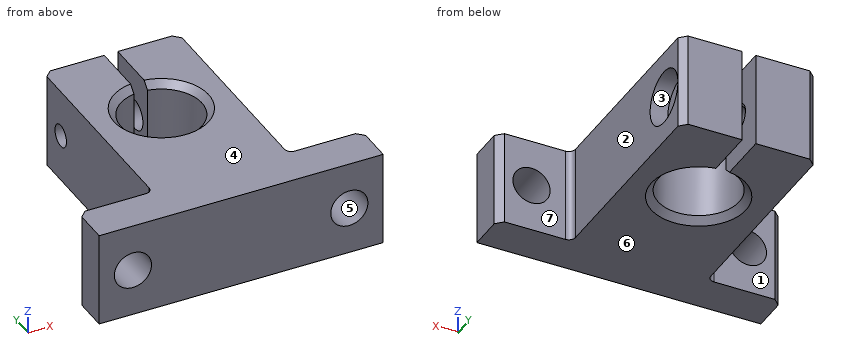
```python
from build123d import *

# Parameters (mm, degrees)
ESTRUSIONE_ESTRUSIONE2_DEPTH                         = 14
FORO_5_5_5_5_3_D                                     = 5.5
FORO_LAMATO_PER_VITE_M4_A_TESTA_CILINDRI_D           = 4.5
FORO_LAMATO_PER_VITE_M4_A_TESTA_CILINDRI_DEPTH       = 9
FORO_LAMATO_PER_VITE_M4_A_TESTA_CILINDRI_CBORE_D     = 8
FORO_LAMATO_PER_VITE_M4_A_TESTA_CILINDRI_CBORE_DEPTH = 2.6
FORO_FILETTATO_M4_1_D                                = 3.3
FORO_FILETTATO_M4_1_CSINK_D                          = 4.05
FORO_FILETTATO_M4_1_CSINK_ANGLE                      = 120
RACCORDO1_R                                          = 1
SMUSSO1_SIZE                                         = 1


with BuildPart() as part:
    # Schizzo10 → Estrusione-Estrusione2 (new body)
    with BuildSketch(Plane.XY):
        with BuildLine():
            Line((21, 0), (-21, 0))
            Line((-21, 0), (-21, 6))
            Line((-21, 6), (-10, 6))
            Line((-10, 6), (-10, 37.5))
            Line((-10, 37.5), (-1, 37.5))
            Line((-1, 37.5), (-1, 28.916079783))
            ThreePointArc((-1, 28.916079783), (0, 17), (1, 28.916079783))
            Line((1, 28.916079783), (1, 37.5))
            Line((1, 37.5), (10, 37.5))
            Line((10, 37.5), (10, 6))
            Line((10, 6), (21, 6))
            Line((21, 6), (21, 0))
        make_face()
    extrude(amount=ESTRUSIONE_ESTRUSIONE2_DEPTH)

    # Foro Ø5.5 (5.5)-3 (through all)
    with Locations(Plane(origin=(0, 6, 0), x_dir=(1, 0, 0), z_dir=(0, 1, 0))):
        with Locations((-16, -7), (16, -7)):
            Hole(FORO_5_5_5_5_3_D / 2)

    # Foro lamato per Vite M4 a testa cilindrica piana-1
    with Locations(Plane(origin=(10, 0, 0), x_dir=(0, 0, -1), z_dir=(1, 0, 0))):
        with Locations((-7, 32.5)):
            CounterBoreHole(FORO_LAMATO_PER_VITE_M4_A_TESTA_CILINDRI_D / 2, FORO_LAMATO_PER_VITE_M4_A_TESTA_CILINDRI_CBORE_D / 2, FORO_LAMATO_PER_VITE_M4_A_TESTA_CILINDRI_CBORE_DEPTH, depth=FORO_LAMATO_PER_VITE_M4_A_TESTA_CILINDRI_DEPTH)

    # Foro filettato M4-1 (through all)
    with Locations(Plane(origin=(-1, 0, 0), x_dir=(0, 0, -1), z_dir=(1, 0, 0))):
        with Locations((-7, 32.5)):
            CounterSinkHole(FORO_FILETTATO_M4_1_D / 2, FORO_FILETTATO_M4_1_CSINK_D / 2, counter_sink_angle=FORO_FILETTATO_M4_1_CSINK_ANGLE)

    # Raccordo1
    raccordo1_edges = [part.edges().sort_by_distance(p)[0] for p in [
        (10, 6, 7),
        (-10, 6, 7),
    ]]
    fillet(raccordo1_edges, radius=RACCORDO1_R)

    # Smusso1
    smusso1_edges = [part.edges().sort_by_distance(p)[0] for p in [
        (0, 17, 0),
        (10, 37.5, 7),
        (21, 6, 7),
        (-21, 6, 7),
        (-10, 37.5, 7),
        (0, 17, 14),
    ]]
    chamfer(smusso1_edges, length=SMUSSO1_SIZE - 0.0001)  # a hair under: the kernel refuses the full size


solid = part.part
```
Geometry check sheet. Reference: the model listing, model coordinates, mm. Face numbers are marked on the shaded views. A direction names the side the tool comes from. Give positions to 0.01 mm unless a question says otherwise; leave off trailing zeros. Loops run counter-clockwise (first coordinate to the right, second up) from the corner with the lowest first, then second, coordinate; pieces in that order, holes last. Notation, with made-up numbers: M -13,20.25 L -7,20.25 A16 ccw -7,25.25 Z; hole C -34,53 d3. An arc over 180 degrees is marked long. Write item = value, one per line.
(1) Sectioned sample at A-A, the plane y = 23. Record the cut outline in (x, z).
Answer below:
outline = M -10,0 L -7,0 L -6,1 L -6,13 L -7,14 L -10,14 Z; M 6,1 L 7,0 L 10,0 L 10,14 L 7,14 L 6,13 Z
(2) Sectioned sample at B-B, the plane z = 2. Record the cut outline in (x, y), plus the area to 3 significant figures.
Answer below:
outline = M -21,0 L 21,0 L 21,5 L 20,6 L 11,6 A1 cw 10,7 L 10,36.5 L 9,37.5 L 1,37.5 L 1,28.92 A6 cw long -1,28.92 L -1,37.5 L -9,37.5 L -10,36.5 L -10,7 A1 cw -11,6 L -20,6 L -21,5 Z
area = 750 mm2
(3) Gauge pin test, flat ends, axial feed: pin 1 Ø4 at (y, z) = (32.5, 7) entering from -X; pin 2 Ø2.5 at (x, z) = (-17, 5) entering from +Y. Record the tip position at first contact, or that the pin passes through.
Answer below:
pin_1 = -10
pin_2 = 6
(4) Material ranges on line 1 (Y direction, x = -7.75, z = 7); line 2 (X direction, y = 7, z = 3); line 3 (Y direction, x = 11, z = 4.5), recorded low to high. Write a range as [from, to].
Answer below:
line_1 = [0, 30.85], [34.15, 37.5]
line_2 = [-10, 10]
line_3 = [0, 6]
(5) Sectioned sample at C-C, the plane x = -7.5. Record the cut outline in (y, z).
Answer below:
outline = M 0,0 L 37.5,0 L 37.5,14 L 0,14 Z; hole C 32.5,7 d3.3
(6) Release check for a two-part mould opening along Z. For the marked faces 5, 6 and 7 record: released by +Z, released by -Z, zero draft, split by the parting line, or undercut.
Answer below:
face_5 = undercut
face_6 = released by -Z
face_7 = zero draft
(7) Sectioned sample at D-D, the plane x = 18. Record the cut outline in (y, z), plus the area to 3 significant figures.
Answer below:
outline = M 0,0 L 6,0 L 6,5.11 L 0,5.11 Z; M 0,8.89 L 6,8.89 L 6,14 L 0,14 Z
area = 61.4 mm2
(8) Tool access check on the marked faces 1, 2, 3 and 4. Record the directions out of +Z, -Z, +X, -X, +Y, -Y that give a thin tool (end or side, any length) a straight path to the whole face; none if there is none.
Answer below:
face_1 = +Z, -Z, -X, +Y
face_2 = +Z, -Z, +X, +Y
face_3 = +X
face_4 = +Z, +X, -X, +Y, -Y
